from build123d import *

# Parameters (mm, degrees)
SKETCH1_R           = 1.2
SKETCH1_R_2         = 4.4
BOSS_EXTRUDE1_DEPTH = 46
SKETCH4_W           = 38
SKETCH4_H           = 30
CUT_EXTRUDE1_DEPTH  = 46


with BuildPart() as part:
    # Sketch1 → Boss-Extrude1 (new body)
    with BuildSketch(Plane.XY):
        with BuildLine():
            Line((8.443747687, 35.125), (-8.876760389, 5.125))
            ThreePointArc((-8.876760389, 5.125), (-5.125, -8.876760389), (8.876760389, -5.125))
            Line((8.876760389, -5.125), (23.238348335, 19.75))
            Line((23.238348335, 19.75), (62.320508076, 19.75))
            Line((62.320508076, 19.75), (62.320508076, 40.25))
            Line((62.320508076, 40.25), (17.320508076, 40.25))
            Line((17.320508076, 40.25), (8.443747687, 35.125))
        make_face()
        with Locations((0, -8)):
            Circle(SKETCH1_R, mode=Mode.SUBTRACT)
        Circle(SKETCH1_R_2, mode=Mode.SUBTRACT)
        with Locations((8, 0)):
            Circle(SKETCH1_R, mode=Mode.SUBTRACT)
        with Locations((-8, 0)):
            Circle(SKETCH1_R, mode=Mode.SUBTRACT)
        with Locations((0, 8)):
            Circle(SKETCH1_R, mode=Mode.SUBTRACT)
    extrude(amount=-BOSS_EXTRUDE1_DEPTH)

    # Sketch4 → Cut-Extrude1 (cut)
    with BuildSketch(Plane(origin=(-8.876760389, 5.125, 0), x_dir=(0, 0, 1), z_dir=(-0.8660254037844382, 0.5000000000000009, 0))):
        with Locations((-23, 4.75)):
            Rectangle(SKETCH4_W, SKETCH4_H)
    extrude(amount=-CUT_EXTRUDE1_DEPTH, mode=Mode.SUBTRACT)


solid = part.part
Geometry: final body of the model. Coordinates: model frame, mm. A direction names the side the tool comes from. Round coordinates to 2 decimals unless told otherwise and drop trailing zeros. Loops run counter-clockwise (first coordinate to the right, second up) from the corner with the lowest first, then second, coordinate; pieces in that order, holes last.
Q1. Pin query (flat end, axial travel): P1, Ø3, axis at x = 2, z = -31.5, coming from the -Y side; P2, Ø1.9, axis at x = 0, y = -8, coming from the -Z side; P3, Ø12, axis at x = 2, z = -20.5, coming from the -Y side; P4, Ø3, axis at y = 26, z = -15.5, coming from the -X side. Return the tip coordinate at first contact, or that it passes through.
Q2. Section B-B on y = 10. Return loops of the section in (x, z), plus the area to 3 significant figures.
Q3. Pull-direction query (Z, two-part tool) for faces 1 (the flat face through (12.9, 37.7, -22.7)), 2 (the flat face through (26, 21, -46)), 3 (the flat face through (9.751, 17.176, -23.266)); classes: released by +Z, released by -Z, zero draft, split by the parting line, or undercut.
Q4. Material intervals for L1, parallel to Z at x = -4.5, y = 8.5; L2, parallel to Y at x = -8, z = -44; L3, parallel to Y at x = 8, z = -44.85, sorted ascending.
Q5. Access query for faces 4 (the flat face through (4, 7, -4)), 5 (the flat face through (62.321, 30, -23)), 6 (the flat face through (43, 19.75, -23)). Directions: +Z, -Z, +X, -X, +Y, -Y. A direction counts if a zero-diameter tool reaches every point of the face in a straight line with its end or side. Return the directions, or none.
Q6. Section A-A on x = -8. Return loops of the section in (y, z).
Q7. Section D-D on y = -8. Return loops of the section in (x, z), plus the area to 3 significant figures.
Evaluation:
1. P1: stops at y = 20.78
1. P2: passes through
1. P3: stops at y = 18.19
1. P4: stops at x = 2.31
2. outline: (-6.06, -46) - (17.61, -46) - (17.61, -42) - (-6.06, -42) - close; (-6.06, -4) - (17.61, -4) - (17.61, 0) - (-6.06, 0) - close
2. area: 189 mm2
3. face 1: zero draft
3. face 2: released by -Z
3. face 3: undercut
4. L1: z = -46 to -42, -4 to 0
4. L2: y = -6.41 to -1.2, 1.2 to 6.64
4. L3: y = -6.41 to -1.2, 1.2 to 34.36
5. face 4: -X, -Y
5. face 5: +Z, -Z, +X, +Y, -Y
5. face 6: +Z, -Z, +X, -Y
6. outline: (-6.41, -46) - (-1.2, -46) - (-1.2, -42) - (-6.41, -42) - close; (-6.41, -4) - (-1.2, -4) - (-1.2, 0) - (-6.41, 0) - close; (1.2, -46) - (6.64, -46) - (6.64, -42) - (1.2, -42) - close; (1.2, -4) - (6.64, -4) - (6.64, 0) - (1.2, 0) - close
7. outline: (-6.41, -46) - (-1.2, -46) - (-1.2, -42) - (-6.41, -42) - close; (-6.41, -4) - (-1.2, -4) - (-1.2, 0) - (-6.41, 0) - close; (1.2, -46) - (6.41, -46) - (6.41, -42) - (1.2, -42) - close; (1.2, -4) - (6.41, -4) - (6.41, 0) - (1.2, 0) - close
7. area: 83.3 mm2
